Print and shaded views of the part. All mm, measured from the part's lowest x, y and z. Round coordinates to 2 decimals unless told otherwise and drop trailing zeros. Loops run counter-clockwise (first coordinate to the right, second up) from the corner with the lowest first, then second, coordinate; pieces in that order, holes last. Notation, with made-up numbers: (82.5, 47) - (100.5, 47) arc R26 ccw to (100.5, 74) - close; hole circle Ø8 at (-9, 2.25). An arc over 180 degrees is marked (long way). Answer as a JSON object with one key per item and string values.
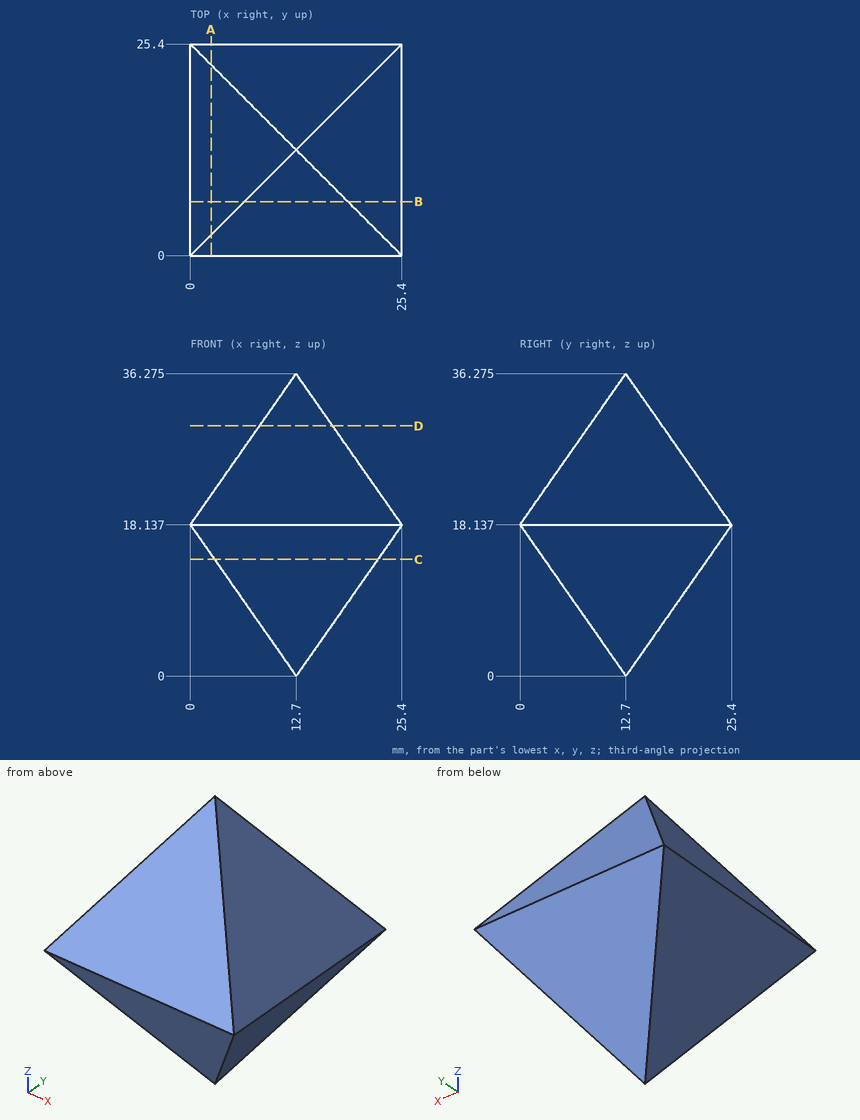
1) Probe probe 1 along X at (y, z) = (20, 12.5); probe 2 along Y at (x, z) = (17.5, 21.5) (1 decimal); probe 3 along Z at (x, y) = (13.5, 8.75) (1 decimal). List the from-to ranges inside material, lowest first.
Values follow:
{"probe 1": "3.95 to 21.45", "probe 2": "2.4 to 23", "probe 3": "5.6 to 30.6"}
2) Slice it at D-D on z = 30. List the corners of the cut face in (x, y).
Values follow:
{"outline": "(8.31, 8.31) - (17.09, 8.31) - (17.09, 17.09) - (8.31, 17.09) - close"}
3) Slice it at B-B on y = 6.5. List the corners of the cut face in (x, z) (1 decimal).
Values follow:
{"outline": "(0, 18.1) - (6.5, 8.9) - (18.9, 8.9) - (25.4, 18.1) - (18.9, 27.4) - (6.5, 27.4) - close"}
4) Slice it at A-A on x = 2.5. List the corners of the cut face in (y, z).
Values follow:
{"outline": "(0, 18.14) - (2.5, 14.57) - (22.9, 14.57) - (25.4, 18.14) - (22.9, 21.71) - (2.5, 21.71) - close"}
5) Drop flat-ended pins along their axis: P1, Ø4, axis at x = 8.5, y = 19, coming from the -Z side; P2, Ø2, axis at y = 16, z = 7, coming from the +X side; P3, Ø12, axis at y = 5.5, z = 10.5, coming from the -X side. Give the stop position or say it passes through.
Values follow:
{"P1": "z = 6.14", "P2": "x = 18.3", "P3": "x = 1.15"}
6) Slice it at C-C on z = 14. List the corners of the cut face in (x, y), then the cut area to 3 significant figures.
Values follow:
{"outline": "(2.9, 2.9) - (22.5, 2.9) - (22.5, 22.5) - (2.9, 22.5) - close", "area": "384 mm²"}
